```python
from build123d import *

# Parameters (mm, degrees)
SKETCH3_BASE_W      = 8.5
SKETCH3_BASE_H      = 8.5
BOSS_EXTRUDE1_DEPTH = 6
SKETCH5_INSERT_R    = 3.825
BOSS_EXTRUDE2_DEPTH = 2
SKETCH6_HOLE_R      = 1.85
CUT_EXTRUDE1_DEPTH  = 9
FILLET1_R           = 1
FILLET2_R           = 1
FILLET3_R           = 0.2


with BuildPart() as part:
    # Sketch3 Base → Boss-Extrude1 (new body)
    with BuildSketch(Plane(origin=(0, 0, 0), x_dir=(1, 0, 0), z_dir=(0, 1, 0))):
        Rectangle(SKETCH3_BASE_W, SKETCH3_BASE_H)
    extrude(amount=BOSS_EXTRUDE1_DEPTH)

    # Sketch5 Insert → Boss-Extrude2 (add)
    with BuildSketch(Plane(origin=(0, 6, 0), x_dir=(1, 0, 0), z_dir=(0, 1, 0))):
        with Locations(Location((0, 0, 0), (0, 0, 270))):  # turned: the seam where the file's is
            Circle(SKETCH5_INSERT_R)
    extrude(amount=BOSS_EXTRUDE2_DEPTH)

    # Sketch6 Hole → Cut-Extrude1 (cut, through all)
    with BuildSketch(Plane(origin=(0, 8, 0), x_dir=(1, 0, 0), z_dir=(0, 1, 0))):
        with Locations(Location((0, 0, 0), (0, 0, 270))):  # turned: the seam where the file's is
            Circle(SKETCH6_HOLE_R)
    extrude(amount=-CUT_EXTRUDE1_DEPTH, mode=Mode.SUBTRACT)

    # Fillet1
    fillet1_edges = [part.edges().sort_by_distance(p)[0] for p in [
        (4.25, 3, -4.25),
        (4.25, 3, 4.25),
        (-4.25, 3, 4.25),
    ]]
    fillet(fillet1_edges, radius=FILLET1_R)

    # Fillet2
    fillet2_edges = [part.edges().sort_by_distance(p)[0] for p in [
        (-4.25, 3, -4.25),
    ]]
    fillet(fillet2_edges, radius=FILLET2_R)

    # Fillet3
    fillet3_edges = [part.edges().sort_by_distance(p)[0] for p in [
        (0, 8, -3.825),
    ]]
    fillet(fillet3_edges, radius=FILLET3_R)


solid = part.part
```
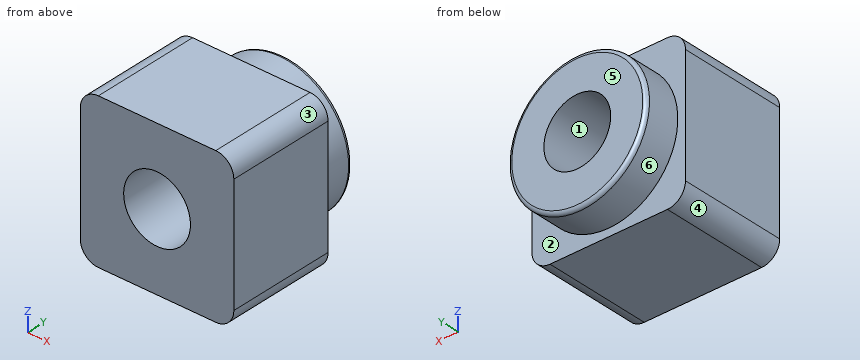
Geometry check sheet. Reference: the model listing, model coordinates, mm. Face numbers are marked on the shaded views. A direction names the side the tool comes from. Round coordinates to 2 decimals unless told otherwise and drop trailing zeros. Order: outer loops, then holes, each group sorted by start corner. A loop starts at its lowest first (then second) coordinate and runs counter-clockwise, first axis right, second up. Notation, with made-up numbers: (30, 30) -> (52, 30) arc R18 ccw to (52, 42) -> close; hole circle Ø1 at (62.25, 26). An arc over 180 degrees is marked (long way). Return JSON: item names as keys, results as strings. Group by question number.
Q1. Tool access check on the marked faces 5 and 6. Record the directions out of +Z, -Z, +X, -X, +Y, -Y that give a thin tool (end or side, any length) a straight path to the whole face; none if there is none.
Q2. Material ranges on probe 1 along X at (y, z) = (3, 0); probe 2 along Y at (x, z) = (3.75, 1.25); probe 3 along Z at (x, y) = (1.25, 7.5), recorded low to high. Write a range as from..to.
Q3. Section check C-C, the plane y = 4.75. Record the boundary of the cut face in (x, z).
Q4. Release check for a two-part mould opening along Z. For the marked faces 1, 2, 3 and 4 record: released by +Z, released by -Z, zero draft, split by the parting line, or undercut.
Q5. Section check A-A, the plane z = 0. Record the boundary of the cut face in (x, y) (3 decimals).
Q6. Section check B-B, the plane x = 0. Record the boundary of the cut face in (y, z) (3 decimals), plus the area to 3 significant figures.
Numbers:
{
 "1": {"face 5": "+Z, -Z, +X, -X, +Y", "face 6": "+Y"},
 "2": {"probe 1": "-4.25..-1.85, 1.85..4.25", "probe 2": "0..6", "probe 3": "-3.61..-1.36, 1.36..3.61"},
 "3": {"outline": "(-4.25, -3.25) arc R1 ccw to (-3.25, -4.25) -> (3.25, -4.25) arc R1 ccw to (4.25, -3.25) -> (4.25, 3.25) arc R1 ccw to (3.25, 4.25) -> (-3.25, 4.25) arc R1 ccw to (-4.25, 3.25) -> close; hole circle Ø3.7 at (0, 0)"},
 "4": {"face 1": "undercut", "face 2": "zero draft", "face 3": "released by +Z", "face 4": "released by -Z"},
 "5": {"outline": "(-4.25, 0) -> (-1.85, 0) -> (-1.85, 8) -> (-3.625, 8) arc R0.2 ccw to (-3.825, 7.8) -> (-3.825, 6) -> (-4.25, 6) -> close; (1.85, 0) -> (4.25, 0) -> (4.25, 6) -> (3.825, 6) -> (3.825, 7.8) arc R0.2 ccw to (3.625, 8) -> (1.85, 8) -> close"},
 "6": {"outline": "(0, -4.25) -> (6, -4.25) -> (6, -3.825) -> (7.8, -3.825) arc R0.2 ccw to (8, -3.625) -> (8, -1.85) -> (0, -1.85) -> close; (0, 1.85) -> (8, 1.85) -> (8, 3.625) arc R0.2 ccw to (7.8, 3.825) -> (6, 3.825) -> (6, 4.25) -> (0, 4.25) -> close", "area": "36.7 mm^2"}
}
